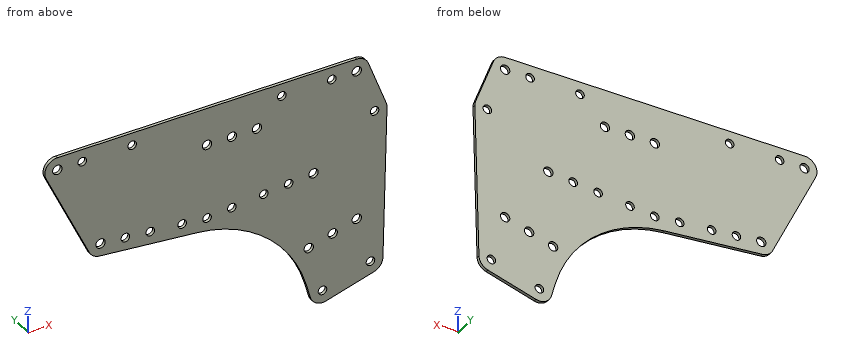
```python
from build123d import *

# Parameters (mm, degrees)
SKETCH1_R           = 2.38125
SKETCH1_R_2         = 2.1828125
BOSS_EXTRUDE1_DEPTH = 1.5875


with BuildPart() as part:
    # Sketch1 → Boss-Extrude1 (new body)
    with BuildSketch(Plane(origin=(0, 0, 0), x_dir=(1, 0, 0), z_dir=(0, 1, 0))):
        with BuildLine():
            Line((0, -6.35), (152.4, -6.35))
            ThreePointArc((152.4, -6.35), (156.001136223, -5.230135553), (158.332104124, -2.265533197))
            Line((158.332104124, -2.265533197), (167.394236912, 21.462883297))
            ThreePointArc((167.394236912, 21.462883297), (167.721572666, 22.659813472), (167.809879929, 23.897550265))
            Line((167.809879929, 23.897550265), (165.742716066, 101.480125789))
            ThreePointArc((165.742716066, 101.480125789), (164.41446111, 105.200361917), (161.143711156, 107.415449457))
            Line((161.143711156, 107.415449457), (136.725881406, 114.410418382))
            ThreePointArc((136.725881406, 114.410418382), (131.897183415, 113.859011684), (128.872681737, 110.054703175))
            Line((128.872681737, 110.054703175), (126.704453603, 102.48591681))
            ThreePointArc((126.704453603, 102.48591681), (106.178087881, 71.080346093), (71.506985471, 56.743114162))
            Line((71.506985471, 56.743114162), (21.41726751, 52.111153689))
            ThreePointArc((21.41726751, 52.111153689), (18.377117757, 51.001852249), (16.278461735, 48.53837846))
            Line((16.278461735, 48.53837846), (-5.723516399, 2.750247267))
            ThreePointArc((-5.723516399, 2.750247267), (-5.375247443, -3.380712192), (0, -6.35))
        make_face()
        Circle(SKETCH1_R, mode=Mode.SUBTRACT)
        with Locations((22.001978134, 45.788131193)):
            Circle(SKETCH1_R, mode=Mode.SUBTRACT)
        with Locations((76.2, 12.7)):
            Circle(SKETCH1_R, mode=Mode.SUBTRACT)
        with Locations((130.398021866, 45.788131193)):
            Circle(SKETCH1_R, mode=Mode.SUBTRACT)
        with Locations((152.4, 0)):
            Circle(SKETCH1_R, mode=Mode.SUBTRACT)
        with Locations((76.2, 50.8)):
            Circle(SKETCH1_R_2, mode=Mode.SUBTRACT)
        with Locations((63.553955008, 49.630578751)):
            Circle(SKETCH1_R_2, mode=Mode.SUBTRACT)
        with Locations((88.846044992, 49.630578751)):
            Circle(SKETCH1_R_2, mode=Mode.SUBTRACT)
        with Locations((117.751976873, 46.957552442)):
            Circle(SKETCH1_R_2, mode=Mode.SUBTRACT)
        with Locations((105.105931881, 48.126973691)):
            Circle(SKETCH1_R_2, mode=Mode.SUBTRACT)
        with Locations((34.648023127, 46.957552442)):
            Circle(SKETCH1_R_2, mode=Mode.SUBTRACT)
        with Locations((47.294068119, 48.126973691)):
            Circle(SKETCH1_R_2, mode=Mode.SUBTRACT)
        with Locations((152.4, 76.893162268)):
            Circle(SKETCH1_R, mode=Mode.SUBTRACT)
        with Locations((127.982170249, 83.888131193)):
            Circle(SKETCH1_R, mode=Mode.SUBTRACT)
        with Locations((140.191085125, 80.390646731)):
            Circle(SKETCH1_R, mode=Mode.SUBTRACT)
        with Locations((134.977139174, 108.305960944)):
            Circle(SKETCH1_R_2, mode=Mode.SUBTRACT)
        with Locations((159.394968925, 101.310992019)):
            Circle(SKETCH1_R_2, mode=Mode.SUBTRACT)
        with Locations((161.462132788, 23.728416494)):
            Circle(SKETCH1_R_2, mode=Mode.SUBTRACT)
        with Locations((12.7, 0)):
            Circle(SKETCH1_R_2, mode=Mode.SUBTRACT)
        with Locations((38.1, 0)):
            Circle(SKETCH1_R_2, mode=Mode.SUBTRACT)
        with Locations((101.6, 12.7)):
            Circle(SKETCH1_R, mode=Mode.SUBTRACT)
        with Locations((88.9, 12.7)):
            Circle(SKETCH1_R, mode=Mode.SUBTRACT)
        with Locations((139.7, 0)):
            Circle(SKETCH1_R_2, mode=Mode.SUBTRACT)
        with Locations((114.3, 0)):
            Circle(SKETCH1_R_2, mode=Mode.SUBTRACT)
    extrude(amount=BOSS_EXTRUDE1_DEPTH)


solid = part.part
```
Geometry check sheet. Reference: the model listing, model coordinates, mm. Give positions to 0.01 mm unless a question says otherwise; leave off trailing zeros. Write each loop counter-clockwise with the first axis right and the second up, starting at its lowest first coordinate (ties: lowest second). Pieces come first, ordered by that corner, then holes.
1) Material ranges on L1, parallel to Z at x = 139.7, y = 1.1; L2, parallel to Z at x = 152.4, y = 0.6; L3, parallel to X at y = 0.4, z = -12.7, recorded low to high.
2) Section check C-C, the plane z = 0. Record the boundary of the cut face in (x, y), and give its area (3 significant figures).
3) Section check D-D, the plane y = 1.2. State how many separate pieces and enclosed holes the cut face has, and give its area (3 significant figures).
4) Section check B-B, the plane x = 12.7. Record the boundary of the cut face in (y, z).
5) Section check A-A, the plane x = 76. Record the boundary of the cut face in (y, z), and give its area (3 significant figures).
Computed:
1. L1: z = -113.56 to -82.72, -78.06 to -2.18, 2.18 to 6.35
1. L2: z = -109.92 to -79.27, -74.51 to -2.38, 2.38 to 6.35
1. L3: x = -0.94 to 73.82, 78.58 to 86.52, 91.28 to 99.22, 103.98 to 164.05
2. outline: (-6.35, 0) - (-2.38, 0) - (-2.38, 1.59) - (-6.35, 1.59) - close; (2.38, 0) - (10.52, 0) - (10.52, 1.59) - (2.38, 1.59) - close; (14.88, 0) - (35.92, 0) - (35.92, 1.59) - (14.88, 1.59) - close; (40.28, 0) - (112.12, 0) - (112.12, 1.59) - (40.28, 1.59) - close; (116.48, 0) - (137.52, 0) - (137.52, 1.59) - (116.48, 1.59) - close; (141.88, 0) - (150.02, 0) - (150.02, 1.59) - (141.88, 1.59) - close; (154.78, 0) - (159.2, 0) - (159.2, 1.59) - (154.78, 1.59) - close
2. area: 220 mm2
3. separate pieces: 1
3. enclosed holes: 24
3. area: 12,400 mm2
4. outline: (0, -41.09) - (1.59, -41.09) - (1.59, -2.18) - (0, -2.18) - close; (0, 2.18) - (1.59, 2.18) - (1.59, 6.35) - (0, 6.35) - close
5. outline: (0, -57.32) - (1.59, -57.32) - (1.59, -52.97) - (0, -52.97) - close; (0, -48.63) - (1.59, -48.63) - (1.59, -15.07) - (0, -15.07) - close; (0, -10.33) - (1.59, -10.33) - (1.59, 6.35) - (0, 6.35) - close
5. area: 86.6 mm2
